The listing builds one solid part. Answer for the finished solid, in the listing's coordinates (mm). Face numbers are marked on the shaded views. Coordinates: 2 decimals unless noted, no trailing zeros. Order: outer loops, then holes, each group sorted by start corner. A loop starts at its lowest first (then second) coordinate and runs counter-clockwise, first axis right, second up. Notation, with made-up numbers: (78, -6.75) -> (102, -6.75) arc R20 cw to (102, 6.25) -> close; hole circle Ø2 at (16.5, -9.75). An arc over 180 degrees is marked (long way). Answer in a Markdown table with one row per item.
Autodesk Inventor part; units mm, degrees
ref_plane "YZ Plane" through (0, 0, 0) normal (1, 0, 0) x (0, 1, 0)
ref_plane "XZ Plane" through (0, 0, 0) normal (0, 1, 0) x (-1, 0, 0)
ref_plane "XY Plane" through (0, 0, 0) normal (0, 0, 1) x (1, 0, 0)
sketch "Sketch1" plane through (0, 0, 0) normal (0, 1, 0) x (-1, 0, 0)
  circle A0 centre (0, 0) radius 25
  circle A1 centre (0, 0) radius 2.25
  dimension "d0" = 50
  dimension "d1" = 4.5
extrude "Extrusion1" add sketch "Sketch1" along normal blind 4
fillet "Fillet1" radius 2 1 edges at (25, 4, 0)
fillet "Fillet2" radius 2 1 edges at (25, 0, 0)
properties part number "Rotor"
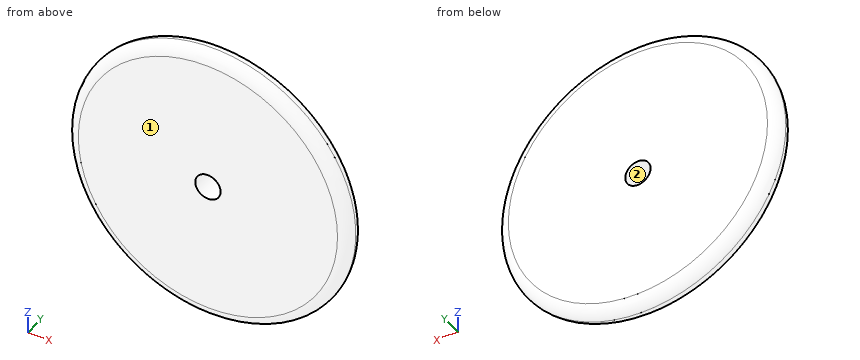
(1) For a pull along Z with two mould halves and no side action, classify the marked faces 1 and 2 as released by +Z, released by -Z, zero draft, split by the parting line, or undercut.
Check values:
| item | result |
|---|---|
| face 1 | zero draft |
| face 2 | undercut |
(2) A cutting plane is placed at C-C, the plane y = 1. Determine the outline of the cut face in (x, z).
Check values:
| item | result |
|---|---|
| outline | circle Ø49.46 at (0, 0); hole circle Ø4.5 at (0, 0) |
(3) Find the intervals of material crossed by line 1 along Z through (x, y) = (0, 2.05); line 2 along Z through (x, y) = (0, 2.85); line 3 along Y through (x, z) = (-21.5, -8.5), in increasing order. Write a range as from..to.
Check values:
| item | result |
|---|---|
| line 1 | -25..-2.25, 2.25..25 |
| line 2 | -24.81..-2.25, 2.25..24.81 |
| line 3 | 0..4 |
